from build123d import *

# Parameters (mm, degrees)
SKETCH_1_W                   = 330
SKETCH_1_H                   = 45
EXTRUDE_1_DEPTH              = 12
HOLE_WIZARD_M5_1_D           = 5.8
HOLE_WIZARD_M5_1_CBORE_D     = 10
HOLE_WIZARD_M5_1_CBORE_DEPTH = 5
SKETCH_4_W                   = 1
SKETCH_4_H                   = 16.5
CUT_EXTRUDE_1_DEPTH          = 334.27016068
SKETCH_5_W                   = 330
SKETCH_5_H                   = 3
EXTRUDE_2_DEPTH              = 1
SKETCH_6_R                   = 11
CUT_EXTRUDE_2_DEPTH          = 334.27016068
SKETCH_9_W                   = 50
SKETCH_9_H                   = 17
CUT_EXTRUDE_5_DEPTH          = 334.27016068
SKETCH_10_W                  = 12
SKETCH_10_H                  = 1.5
CUT_EXTRUDE_6_DEPTH          = 334.27016068
SKETCH_11_R                  = 15
CUT_EXTRUDE_7_DEPTH          = 6
SKETCH_14_R                  = 2.75
CUT_EXTRUDE_8_DEPTH          = 334.27016068
HOLE_WIZARD_M5_2_D           = 5.8
HOLE_WIZARD_M5_2_CBORE_D     = 10
HOLE_WIZARD_M5_2_CBORE_DEPTH = 5


with BuildPart() as part:
    # 草图1 → 凸台-拉伸1 (new body)
    with BuildSketch(Plane.XY):
        with Locations((165, 22.5)):
            Rectangle(SKETCH_1_W, SKETCH_1_H)
    extrude(amount=EXTRUDE_1_DEPTH)

    # M5 六角凹头螺钉的柱形沉头孔1 (through all)
    with Locations(Plane.XY.offset(12)):
        with Locations((10, 24), (50, 24)):
            CounterBoreHole(HOLE_WIZARD_M5_1_D / 2, HOLE_WIZARD_M5_1_CBORE_D / 2, HOLE_WIZARD_M5_1_CBORE_DEPTH)

    # 草图4 → 切除-拉伸1 (cut, through all)
    with BuildSketch(Plane.ZY):
        with Locations((0.5, 36.75)):
            Rectangle(SKETCH_4_W, SKETCH_4_H)
    extrude(amount=-CUT_EXTRUDE_1_DEPTH, mode=Mode.SUBTRACT)

    # 草图5 → 凸台-拉伸2 (add)
    with BuildSketch(Plane(origin=(0, 0, 1), x_dir=(-1, 0, 0), z_dir=(0, 0, -1))):
        with Locations((-165, 43.5)):
            Rectangle(SKETCH_5_W, SKETCH_5_H)
    extrude(amount=EXTRUDE_2_DEPTH)

    # 草图6 → 切除-拉伸2 (cut, through all)
    with BuildSketch(Plane.XY.offset(12)):
        with Locations((165, 22.5)):
            Circle(SKETCH_6_R)
    extrude(amount=-CUT_EXTRUDE_2_DEPTH, mode=Mode.SUBTRACT)

    # 草图9 → 切除-拉伸5 (cut, through all)
    with BuildSketch(Plane.XY.offset(12)):
        with Locations((25, 8.5)):
            Rectangle(SKETCH_9_W, SKETCH_9_H)
        with Locations((305, 8.5)):
            Rectangle(SKETCH_9_W, SKETCH_9_H)
    extrude(amount=-CUT_EXTRUDE_5_DEPTH, mode=Mode.SUBTRACT)

    # 草图10 → 切除-拉伸6 (cut, through all)
    with BuildSketch(Plane.XZ):
        with Locations((146, 11.25)):
            Rectangle(SKETCH_10_W, SKETCH_10_H)
    extrude(amount=-CUT_EXTRUDE_6_DEPTH, mode=Mode.SUBTRACT)

    # 草图11 → 切除-拉伸7 (cut)
    with BuildSketch(Plane(origin=(0, 0, 0), x_dir=(-1, 0, 0), z_dir=(0, 0, -1))):
        with Locations((-165, 22.5)):
            Circle(SKETCH_11_R)
    extrude(amount=-CUT_EXTRUDE_7_DEPTH, mode=Mode.SUBTRACT)

    # 草图14 → 切除-拉伸8 (cut, through all)
    with BuildSketch(Plane.XY.offset(12)):
        with Locations((280, 24)):
            Circle(SKETCH_14_R)
        with Locations((320, 24)):
            Circle(SKETCH_14_R)
    extrude(amount=-CUT_EXTRUDE_8_DEPTH, mode=Mode.SUBTRACT)

    # M5 六角凹头螺钉的柱形沉头孔2 (through all)
    with Locations(Plane(origin=(0, 0, 0), x_dir=(-1, 0, 0), z_dir=(0, 0, -1))):
        with Locations((-146, 6), (-146, 21)):
            CounterBoreHole(HOLE_WIZARD_M5_2_D / 2, HOLE_WIZARD_M5_2_CBORE_D / 2, HOLE_WIZARD_M5_2_CBORE_DEPTH)


solid = part.part
Work out the finished part from the listing and answer in its coordinate system (mm). A direction names the side the tool comes from. Give positions to 0.01 mm unless a question says otherwise; leave off trailing zeros. Loops run counter-clockwise (first coordinate to the right, second up) from the corner with the lowest first, then second, coordinate; pieces in that order, holes last. Notation, with made-up numbers: M 43,15 L 74,15 A15 ccw 74,27 Z; hole C 65,64 d5. An arc over 180 degrees is marked long. Use CSV: the item, a comma, the result in double quotes.
1) Which of the six approach directions +Z, -Z, +X, -X, +Y, -Y give full straight-line access (tool end or side, diameter ignored) to faces 5 (the cylindrical face through (12.307, 19.564, 9.535)), 6 (the flat face through (143.7, 18.8, 5)), 7 (the flat face through (280, 8, 6)), 8 (the flat face through (163, 38, 1))?
Answer:
face 5,"+Z"
face 6,"-Z"
face 7,"+Z, -Z, +X, -Y"
face 8,"-Z, +X, -X"
2) Find section B-B on x = 76. Write down the section's boundary in (y, z), plus the area to 4 significant figures.
Answer:
outline,"M 0,0 L 28.5,0 L 28.5,1 L 42,1 L 42,0 L 45,0 L 45,12 L 0,12 Z"
area,"526.5 mm^2"
3) Given P1, Ø3.5, axis at y = 5, z = 4.5, coming from the -X side; P2, Ø6.5, axis at x = 146, y = 6, coming from the +Z side; P3, Ø6, axis at x = 22, z = 8, coming from the -Y side, each flat-ended and moving along its own axis, determine where each tip first touches the part or whether it passes through.
Answer:
P1,"x = 50"
P2,"z = 10.5"
P3,"y = 17"
4) Consider L1, parallel to X at y = 22.5, z = 2.05; L2, parallel to Y at x = 146, z = 9.35; L3, parallel to Y at x = 165, z = 10.55. Determine where each line is inside the solid, lowest interval first.
Answer:
L1,"0 to 7.52, 12.48 to 47.52, 52.48 to 141.23, 180 to 277.7, 282.3 to 317.7, 322.3 to 330"
L2,"0 to 3.1, 8.9 to 18.1, 23.9 to 45"
L3,"0 to 11.5, 33.5 to 45"
5) Determine the mould class of faces 1 (the flat face through (0, 31, 6)), 2 (the flat face through (12.2, 21.8, 7)), 3 (the flat face through (305, 17, 6)), 4 (the cylindrical face through (282.62, 24.83, 6.08)) for opening direction X: released by +X, released by -X, zero draft, split by the parting line, or undercut.
Answer:
face 1,"released by -X"
face 2,"undercut"
face 3,"zero draft"
face 4,"undercut"
6) Find section A-A on x = 165. Write down the section's boundary in (y, z), plus the area to 4 significant figures.
Answer:
outline,"M 0,0 L 7.5,0 L 7.5,6 L 11.5,6 L 11.5,12 L 0,12 Z; M 33.5,6 L 37.5,6 L 37.5,1 L 42,1 L 42,0 L 45,0 L 45,12 L 33.5,12 Z"
area,"223.5 mm^2"
